```python
from build123d import *

# Parameters (mm, degrees)
F1_DEPTH = 12.5
F2_R     = 9.1118495461
F2_R_2   = 8.7709801572
F3_DEPTH = 13.2479583845


with BuildPart() as f1:
    # F0 (on Right) → F1 (new body, symmetric)
    with BuildSketch(Plane.YZ):
        Polygon((25.6182104349, -14.181278646), (25.6182104349, 26.9834250212), (-8.1956535578, 26.8364101648), (-16.7226195335, 7.8712403774), (-33.9235812426, 7.8712403774), (-33.9235812426, -14.181278646), align=None)
    extrude(amount=F1_DEPTH, both=True)

    # F2 (on Right) → F3 (join, symmetric)
    with BuildSketch(Plane.YZ):
        with Locations((-23.2708677649, -8.7504684925)):
            Circle(F2_R)
        with Locations((13.5083943605, -8.7504684925)):
            Circle(F2_R_2)
    extrude(amount=F3_DEPTH, both=True)


solid = f1.part
```
The listing builds one solid part. Answer for the finished solid, in the listing's coordinates (mm). A direction names the side the tool comes from. Round coordinates to 2 decimals unless told otherwise and drop trailing zeros. Loops run counter-clockwise (first coordinate to the right, second up) from the corner with the lowest first, then second, coordinate; pieces in that order, holes last.
1) A cutting plane is placed at A-A on x = 4.5. Determine the outline of the cut face in (y, z).
Outcome:
outline: (-33.92, -14.18) - (-30.59, -14.18) arc R9.11 ccw to (-15.95, -14.18) - (6.62, -14.18) arc R8.77 ccw to (20.4, -14.18) - (25.62, -14.18) - (25.62, 26.98) - (-8.2, 26.84) - (-16.72, 7.87) - (-33.92, 7.87) - close
2) Given P1, Ø4, axis at x = 3.5, y = 22, coming from the -Z side; P2, Ø10, axis at y = 0, z = -0.5, coming from the -X side; P3, Ø8, axis at x = -0.5, z = 18, coming from the -Y side, each flat-ended and moving along its own axis, determine where each tip first touches the part or whether it passes through.
Outcome:
P1: stops at z = -14.65
P2: stops at x = -12.5
P3: stops at y = -13.97
3) A cutting plane is placed at C-C on y = -22. Determine the outline of the cut face in (x, z).
Outcome:
outline: (-13.25, -17.77) - (13.25, -17.77) - (13.25, 0.27) - (12.5, 0.27) - (12.5, 7.87) - (-12.5, 7.87) - (-12.5, 0.27) - (-13.25, 0.27) - close
4) For faces 4 (the face through (0, -25, 7.871)), 5 (the face through (0, 23, -14.181)), 6 (the face through (0, -33.924, -3)), 7 (the face through (13.248, 13, -9)), 8 (the face through (0, -32, -14.181)), determine the directions among +Z, -Z, +X, -X, +Y, -Y from which every point of the face is accessible in a straight line to the end or side of a thin tool.
Outcome:
face 4: +Z, +X, -X, -Y
face 5: -Z, +X, -X, +Y
face 6: +Z, -Z, +X, -X, -Y
face 7: +Z, -Z, +X, +Y, -Y
face 8: -Z, +X, -X, -Y
5) Consider line 1 (X direction, y = 6.5, z = 3.5); line 2 (Y direction, x = -10.5, z = -15); line 3 (Z direction, x = -9, y = -7). Determine where each line is inside the solid, lowest interval first.
Outcome:
line 1: x = -12.5 to 12.5
line 2: y = -29.9 to -16.64, 7.35 to 19.66
line 3: z = -14.18 to 26.84
6) A cutting plane is placed at D-D on z = -5.5. Determine the outline of the cut face in (x, y).
Outcome:
outline: (-13.25, -31.78) - (-12.5, -31.78) - (-12.5, -33.92) - (12.5, -33.92) - (12.5, -31.78) - (13.25, -31.78) - (13.25, -14.76) - (12.5, -14.76) - (12.5, 5.36) - (13.25, 5.36) - (13.25, 21.65) - (12.5, 21.65) - (12.5, 25.62) - (-12.5, 25.62) - (-12.5, 21.65) - (-13.25, 21.65) - (-13.25, 5.36) - (-12.5, 5.36) - (-12.5, -14.76) - (-13.25, -14.76) - close
7) For a pull along Y with two mould halves and no side action, classify faces 1 (the face through (-13.248, -23, -9)), 2 (the face through (0, -5, -14.181)), 3 (the face through (0.18, -12.4, 17.49)) as released by +Y, released by -Y, zero draft, split by the parting line, or undercut.
Outcome:
face 1: zero draft
face 2: undercut
face 3: released by -Y
8) A cutting plane is placed at B-B on z = -15. Determine the outline of the cut face in (x, y).
Outcome:
outline: (-13.25, -29.9) - (13.25, -29.9) - (13.25, -16.64) - (-13.25, -16.64) - close; (-13.25, 7.35) - (13.25, 7.35) - (13.25, 19.66) - (-13.25, 19.66) - close
